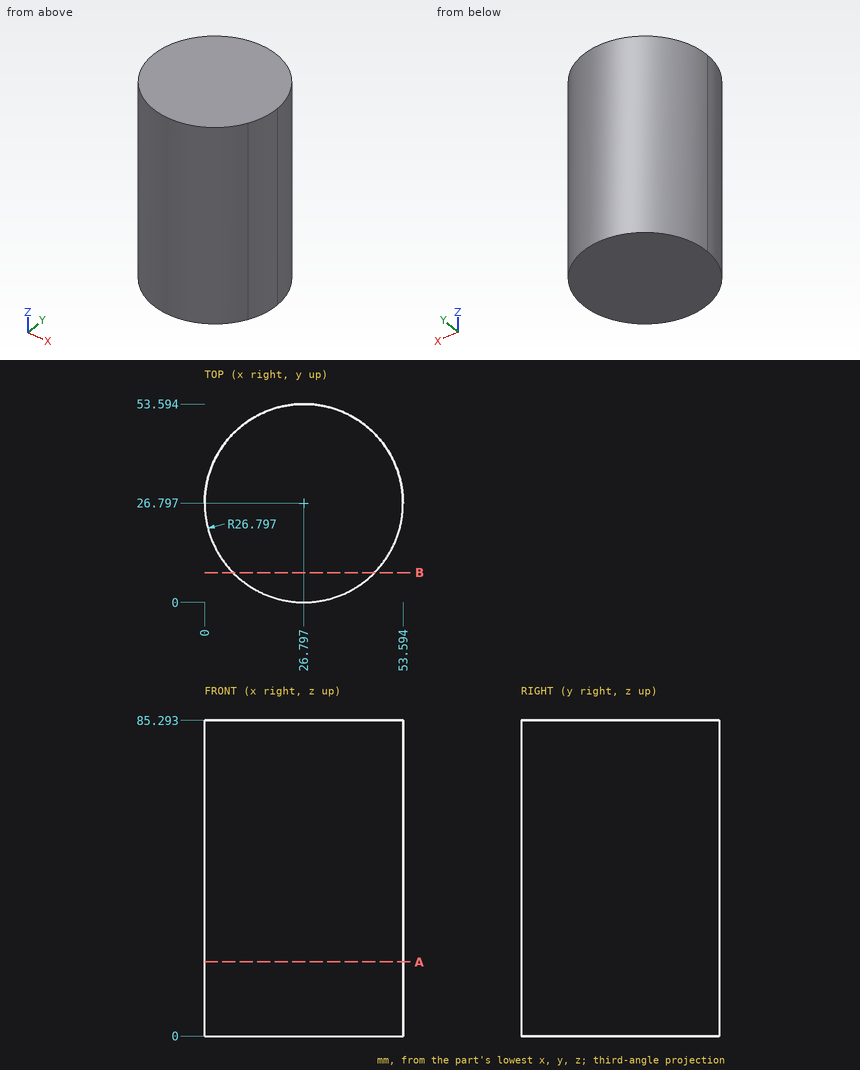
Geometry check sheet. Reference: drawing and pictorial views, mm from the part's lowest x, y, z. Give positions to 0.01 mm unless a question says otherwise; leave off trailing zeros. Write each loop counter-clockwise with the first axis right and the second up, starting at its lowest first coordinate (ties: lowest second). Pieces come first, ordered by that corner, then holes. Notation, with made-up numbers: (-31, 70.25) -> (2, 70.25) arc R30 ccw to (2, 94.25) -> close; hole circle Ø10 at (80.25, 1.25). An arc over 180 degrees is marked (long way). One line per item, written item: value. Start each with the question number.
Item 1: Section check A-A on z = 20. Record the cut outline in (x, y) (1 decimal), then the cut area to 3 significant figures.
Item 2: Gauge pin test, flat ends, axial feed: pin 1 (10 mm diameter, centred on y = 12.5, z = 37, fed in from +X); pin 2 (1.5 mm diameter, centred on y = 48, z = 42.5, fed in from -X); pin 3 (4 mm diameter, centred on y = 33.5, z = 27.5, fed in from +X). Record the tip position at first contact, or that the pin passes through.
Item 3: Section check B-B on y = 8. Record the cut outline in (x, z).
Item 4: Material ranges on probe 1 along X at (y, z) = (26.5, 23.5); probe 2 along X at (y, z) = (5, 20) (1 decimal), recorded low to high. Write a range as from..to.
Results list:
1. outline: (0, 26.8) arc R26.8 ccw to (3.4, 13.8) arc R26.8 ccw to (50.2, 13.8) arc R26.8 ccw to (53.6, 26.8) arc R26.8 ccw to start
1. area: 2,260 mm²
2. pin 1: x = 51.93
2. pin 2: x = 9.48
2. pin 3: x = 53.18
3. outline: (7.7, 0) -> (45.9, 0) -> (45.9, 85.29) -> (7.7, 85.29) -> close
4. probe 1: 0..53.59
4. probe 2: 11.2..42.4
